Source: CAD feature listing. Evaluate the final solid. Frame: model axes, mm. Face numbers are marked on the shaded views. A direction names the side the tool comes from. Coordinates: 2 decimals unless noted, no trailing zeros. Loops run counter-clockwise (first coordinate to the right, second up) from the corner with the lowest first, then second, coordinate; pieces in that order, holes last.
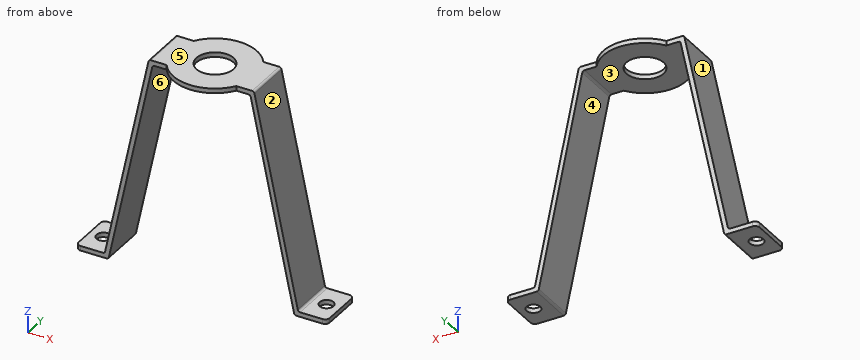
```python
from build123d import *

# Parameters (mm, degrees)
F2_W      = 10
F2_H      = 1
F4_R      = 0.5
F5_R      = 9
F6_DEPTH  = 1
F7_R      = 4
F8_DEPTH  = 1
F9_R      = 1.5
F10_DEPTH = 1
F11_R     = 1


with BuildPart() as f3:
    # F3: sweep along a path in F0
    with BuildLine(Plane.XZ) as f3_path:
        Line((27, 0), (20, 0))
        Line((20, 0), (10.5, 45))
        Line((10.5, 45), (-10.5, 45))
        Line((-10.5, 45), (-20, 0))
        Line((-20, 0), (-27, 0))
    # F2 (on plane+point) → F3 (sweep)
    with BuildSketch(Plane.YZ.offset(27)):
        with Locations((0, 0.5)):
            Rectangle(F2_W, F2_H)
    sweep(path=f3_path.line, transition=Transition.RIGHT)

    # F4
    f4_edges = [f3.edges().sort_by_distance(p)[0] for p in [
        (20.81093, 0, 1),
        (11.31093, 0, 46),
        (-11.31093, 0, 46),
        (-20.81093, 0, 1),
        (20, 0, 0),
        (10.5, 0, 45),
        (-20, 0, 0),
        (-10.5, 0, 45),
    ]]
    fillet(f4_edges, radius=F4_R)

    # F5 (on face) → F6 (join, through all)
    with BuildSketch(Plane.XY.offset(46)):
        Circle(F5_R)
    extrude(amount=-F6_DEPTH)

    # F7 (on face) → F8 (cut, through all)
    with BuildSketch(Plane.XY.offset(46)):
        Circle(F7_R)
    extrude(amount=-F8_DEPTH, mode=Mode.SUBTRACT)

    # F9 (on Top) → F10 (cut, through all)
    with BuildSketch(Plane.XY):
        with Locations((-24, 0)):
            Circle(F9_R)
        with Locations((24, 0)):
            Circle(F9_R)
    extrude(amount=F10_DEPTH, mode=Mode.SUBTRACT)

    # F11
    f11_edges = [f3.edges().sort_by_distance(p)[0] for p in [
        (27, -5, 0.5),
        (27, 5, 0.5),
        (-27, 5, 0.5),
        (-27, -5, 0.5),
    ]]
    fillet(f11_edges, radius=F11_R)


solid = f3.part
```
Q1. Section query B-B on x = 24. Return the cut outline in (y, z).
Q2. Material intervals for line 1 along Z through (x, y) = (-3, 2.75); line 2 along X through (y, z) = (-2.75, 26.5); line 3 along X through (y, z) = (-3, 21), sorted ascending.
Q3. Section query D-D on y = -3. Return the cut outline in (x, z), then the cut area to 3 significant figures.
Q4. Section query A-A on y = 0. Count the separate pieces of the cut face and the enclosed holes in it, then the cut area to 3 significant figures.
Q5. First-contact query: pin 1 Ø5.5 at (x, z) = (-15, 20) entering from +Y; pin 2 Ø20.5 at (x, z) = (-14.5, 28) entering from -Y; pin 3 Ø4.5 at (x, y) = (25.5, 1) entering from +Z. Flat tips, straight axial feed; report the tip coordinate or a pass-through.
Q6. Draft query along X for the marked faces 1, 2, 3 and 4. Return one class per face: released by +X, released by -X, zero draft, split by the parting line, or undercut.
Q7. Section query C-C on z = 10. Return the cut outline in (x, y).
Q8. Reachability of the marked faces 5 and 6 from +Z, -Z, +X, -X, +Y, -Y: full face, straight path, thin tool, end or side. Return the list, or none.
Resolved:
1. outline: (-5, 0) - (-1.5, 0) - (-1.5, 1) - (-5, 1) - close; (1.5, 0) - (5, 0) - (5, 1) - (1.5, 1) - close
2. line 1: z = 45 to 46
2. line 2: x = -15.43 to -14.41, 14.41 to 15.43
2. line 3: x = -16.59 to -15.57, 15.57 to 16.59
3. outline: (-27, 0) - (-20.41, 0) arc R0.5 ccw to (-19.92, 0.4) - (-10.58, 44.6) arc R0.5 cw to (-10.09, 45) - (-2.65, 45) - (-2.65, 46) - (-10.91, 46) arc R0.5 ccw to (-11.39, 45.6) - (-20.73, 1.4) arc R0.5 cw to (-21.22, 1) - (-27, 1) - close; (2.65, 45) - (10.09, 45) arc R0.5 cw to (10.58, 44.6) - (19.92, 0.4) arc R0.5 ccw to (20.41, 0) - (27, 0) - (27, 1) - (21.22, 1) arc R0.5 cw to (20.73, 1.4) - (11.39, 45.6) arc R0.5 ccw to (10.91, 46) - (2.65, 46) - close
3. area: 122 mm2
4. separate pieces: 4
4. enclosed holes: 0
4. area: 113 mm2
5. pin 1: stops at y = 5
5. pin 2: stops at y = -5
5. pin 3: stops at z = 1
6. face 1: released by -X
6. face 2: released by +X
6. face 3: undercut
6. face 4: undercut
7. outline: (-18.91, -5) - (-17.89, -5) - (-17.89, 5) - (-18.91, 5) - close; (17.89, -5) - (18.91, -5) - (18.91, 5) - (17.89, 5) - close
8. face 5: +Z, +X, -X, +Y, -Y
8. face 6: -Z, +Y, -Y
